Geometry check sheet. Reference: the model listing, model coordinates, mm. Round coordinates to 2 decimals unless told otherwise and drop trailing zeros. Order: outer loops, then holes, each group sorted by start corner. A loop starts at its lowest first (then second) coordinate and runs counter-clockwise, first axis right, second up.
(1) Sectioned sample at B-B (z = -23.6). Record the boundary of the cut face in (x, y).
(2) Go/stop test with flat-tipped pins: pin 1 (4 mm diameter, centred on y = 6.5, z = 106, fed in from +X); pin 2 (2.5 mm diameter, centred on y = 4.5, z = -104.5, fed in from -X); pin 3 (1.9 mm diameter, centred on x = 79, y = 3.5, fed in from -Z). Record where each tip stops, or that it passes through.
(3) Sectioned sample at C-C (y = 7.5). Give the number of separate pieces and of enclosed holes in the cut face, plus the area to 3 significant figures.
(4) Sectioned sample at A-A (x = 70). Record the boundary of the cut face in (y, z).
(5) Sectioned sample at D-D (x = -37.5). Record the boundary of the cut face in (y, z), plus the area to 3 significant figures.
(6) Material ranges on line 1 along Z through (x, y) = (23.5, 2.25); line 2 along X through (y, z) = (6.5, 23.6); line 3 along X through (y, z) = (6.5, -100.5), recorded low to high.
from build123d import *

# Parameters (mm, degrees)
SKETCH1_W            = 260
SKETCH1_H            = 200
EXTRUDE1_DEPTH       = 10
SKETCH3_W            = 20
SKETCH3_H            = 10
EXTRUDE2_DEPTH       = 10
M4_CLEARANCE_HOLE1_D = 4.5
EXTRUDE3_DEPTH       = 10
MIRROR2_COPY_1_DEPTH = 10
MIRROR3_COPY_1_DEPTH = 10
MIRROR3_COPY_2_DEPTH = 10
MIRROR3_COPY_3_DEPTH = 10
SKETCH7_W            = 20
SKETCH7_H            = 10
EXTRUDE4_DEPTH       = 10
LPATTERN1_COUNT      = 2
LPATTERN1_PITCH      = 170
LPATTERN1_COUNT_DIR2 = 2
LPATTERN1_PITCH_DIR2 = 210
EXTRUDE5_DEPTH       = 10
MIRROR5_COPY_1_DEPTH = 10
EXTRUDE6_DEPTH       = 10
MIRROR7_COPY_1_DEPTH = 10
SKETCH11_R           = 19.05
SKETCH11_R_2         = 2.75
CUT_EXTRUDE2_DEPTH   = 10


with BuildPart() as part:
    # Sketch1 → Extrude1 (new body)
    with BuildSketch(Plane(origin=(0, 0, 0), x_dir=(1, 0, 0), z_dir=(0, 1, 0))):
        Rectangle(SKETCH1_W, SKETCH1_H)
    extrude(amount=EXTRUDE1_DEPTH)

    # Sketch3 → Extrude2 (cut)
    with BuildSketch(Plane(origin=(0, 10, 0), x_dir=(1, 0, 0), z_dir=(0, 1, 0))):
        with Locations((-105, 45)):
            Rectangle(SKETCH3_W, SKETCH3_H)
        with Locations((105, 45)):
            Rectangle(SKETCH3_W, SKETCH3_H)
        with Locations((-65, 45)):
            Rectangle(SKETCH3_W, SKETCH3_H)
        with Locations((65, 45)):
            Rectangle(SKETCH3_W, SKETCH3_H)
    extrude(amount=-EXTRUDE2_DEPTH, mode=Mode.SUBTRACT)

    # M4 Clearance Hole1 (through all)
    with Locations(Plane(origin=(0, 10, 0), x_dir=(1, 0, 0), z_dir=(0, 1, 0))):
        with Locations((-85, 45), (85, 45)):
            Hole(M4_CLEARANCE_HOLE1_D / 2)

    # Sketch6 → Extrude3 (cut)
    with BuildSketch(Plane(origin=(0, 10, 0), x_dir=(1, 0, 0), z_dir=(0, 1, 0))):
        with BuildLine():
            Line((-113.5, 50), (-115, 50))
            Line((-115, 50), (-115, 48.5))
            ThreePointArc((-115, 48.5), (-116.060660172, 51.060660172), (-113.5, 50))
        make_face()
        with BuildLine():
            Line((-113.5, 40), (-115, 40))
            Line((-115, 40), (-115, 41.5))
            ThreePointArc((-115, 41.5), (-116.060660172, 38.939339828), (-113.5, 40))
        make_face()
    extrude3 = extrude(amount=-EXTRUDE3_DEPTH, mode=Mode.SUBTRACT)

    # Mirror1: Extrude3 across plane
    add(extrude3.mirror(Plane(origin=(-105, 0, 0), x_dir=(0, 0, 1), z_dir=(1, 0, 0))), mode=Mode.SUBTRACT)

    # Mirror2: Extrude3 across plane
    add(extrude3.mirror(Plane.ZY.offset(85)), mode=Mode.SUBTRACT)

    # Mirror2 copy 1 sketch → Mirror2 copy 1 (cut)
    with BuildSketch(Plane(origin=(40, 10, 0), x_dir=(1, 0, 0), z_dir=(0, 1, 0))):
        with BuildLine():
            Line((-113.5, 50), (-115, 50))
            Line((-115, 50), (-115, 48.5))
            ThreePointArc((-115, 48.5), (-116.060660172, 51.060660172), (-113.5, 50))
        make_face()
        with BuildLine():
            Line((-113.5, 40), (-115, 40))
            Line((-115, 40), (-115, 41.5))
            ThreePointArc((-115, 41.5), (-116.060660172, 38.939339828), (-113.5, 40))
        make_face()
    extrude(amount=-MIRROR2_COPY_1_DEPTH, mode=Mode.SUBTRACT)

    # Mirror3: Extrude3 across plane
    add(extrude3.mirror(Plane(origin=(0, 0, 0), x_dir=(0, 0, 1), z_dir=(1, 0, 0))), mode=Mode.SUBTRACT)

    # Mirror3 copy 1 sketch → Mirror3 copy 1 (cut)
    with BuildSketch(Plane(origin=(210, 10, 0), x_dir=(1, 0, 0), z_dir=(0, 1, 0))):
        with BuildLine():
            Line((-113.5, 50), (-115, 50))
            Line((-115, 50), (-115, 48.5))
            ThreePointArc((-115, 48.5), (-116.060660172, 51.060660172), (-113.5, 50))
        make_face()
        with BuildLine():
            Line((-113.5, 40), (-115, 40))
            Line((-115, 40), (-115, 41.5))
            ThreePointArc((-115, 41.5), (-116.060660172, 38.939339828), (-113.5, 40))
        make_face()
    extrude(amount=-MIRROR3_COPY_1_DEPTH, mode=Mode.SUBTRACT)

    # Mirror3 copy 2 sketch → Mirror3 copy 2 (cut)
    with BuildSketch(Plane(origin=(170, 10, 0), x_dir=(1, 0, 0), z_dir=(0, 1, 0))):
        with BuildLine():
            Line((-113.5, 50), (-115, 50))
            Line((-115, 50), (-115, 48.5))
            ThreePointArc((-115, 48.5), (-116.060660172, 51.060660172), (-113.5, 50))
        make_face()
        with BuildLine():
            Line((-113.5, 40), (-115, 40))
            Line((-115, 40), (-115, 41.5))
            ThreePointArc((-115, 41.5), (-116.060660172, 38.939339828), (-113.5, 40))
        make_face()
    extrude(amount=-MIRROR3_COPY_2_DEPTH, mode=Mode.SUBTRACT)

    # Mirror3 copy 3 sketch → Mirror3 copy 3 (cut)
    with BuildSketch(Plane(origin=(-40, 10, 0), x_dir=(-1, 0, 0), z_dir=(0, 1, 0))):
        with BuildLine():
            Line((-113.5, -50), (-115, -50))
            Line((-115, -50), (-115, -48.5))
            ThreePointArc((-115, -48.5), (-116.060660172, -51.060660172), (-113.5, -50))
        make_face()
        with BuildLine():
            Line((-113.5, -40), (-115, -40))
            Line((-115, -40), (-115, -41.5))
            ThreePointArc((-115, -41.5), (-116.060660172, -38.939339828), (-113.5, -40))
        make_face()
    extrude(amount=-MIRROR3_COPY_3_DEPTH, mode=Mode.SUBTRACT)

    # Sketch7 → Extrude4 (add)
    with BuildSketch(Plane(origin=(0, 10, 0), x_dir=(1, 0, 0), z_dir=(0, 1, 0))):
        with Locations((-105, -105)):
            Rectangle(SKETCH7_W, SKETCH7_H)
        with Locations((-65, -105)):
            Rectangle(SKETCH7_W, SKETCH7_H)
    extrude4 = extrude(amount=-EXTRUDE4_DEPTH)

    # LPattern1: Extrude4 2 × 2
    with Locations(*[(i * LPATTERN1_PITCH, 0, -j * LPATTERN1_PITCH_DIR2) for i in range(LPATTERN1_COUNT) for j in range(LPATTERN1_COUNT_DIR2) if (i, j) != (0, 0)]):
        add(extrude4)

    # Sketch8 → Extrude5 (cut)
    with BuildSketch(Plane(origin=(0, 10, 0), x_dir=(1, 0, 0), z_dir=(0, 1, 0))):
        with BuildLine():
            Line((-116.5, -100), (-115, -100))
            Line((-115, -100), (-115, -101.5))
            ThreePointArc((-115, -101.5), (-113.939339828, -98.939339828), (-116.5, -100))
        make_face()
        with BuildLine():
            Line((-95, -101.5), (-95, -100))
            Line((-95, -100), (-93.5, -100))
            ThreePointArc((-93.5, -100), (-96.060660172, -98.939339828), (-95, -101.5))
        make_face()
        with BuildLine():
            Line((-75, -100), (-75, -101.5))
            ThreePointArc((-75, -101.5), (-73.939339828, -98.939339828), (-76.5, -100))
            Line((-76.5, -100), (-75, -100))
        make_face()
        with BuildLine():
            Line((-55, -101.5), (-55, -100))
            Line((-55, -100), (-53.5, -100))
            ThreePointArc((-53.5, -100), (-56.060660172, -98.939339828), (-55, -101.5))
        make_face()
    extrude5 = extrude(amount=-EXTRUDE5_DEPTH, mode=Mode.SUBTRACT)

    # Mirror4: Extrude5 across plane
    add(extrude5.mirror(Plane(origin=(0, 0, 0), x_dir=(0, 0, 1), z_dir=(1, 0, 0))), mode=Mode.SUBTRACT)

    # Mirror5: Extrude5 across plane
    add(extrude5.mirror(Plane.XY), mode=Mode.SUBTRACT)

    # Mirror5 copy 1 sketch → Mirror5 copy 1 (cut)
    with BuildSketch(Plane(origin=(0, 10, 0), x_dir=(-1, 0, 0), z_dir=(0, 1, 0))):
        with BuildLine():
            Line((-116.5, -100), (-115, -100))
            Line((-115, -100), (-115, -101.5))
            ThreePointArc((-115, -101.5), (-113.939339828, -98.939339828), (-116.5, -100))
        make_face()
        with BuildLine():
            Line((-95, -101.5), (-95, -100))
            Line((-95, -100), (-93.5, -100))
            ThreePointArc((-93.5, -100), (-96.060660172, -98.939339828), (-95, -101.5))
        make_face()
        with BuildLine():
            Line((-75, -100), (-75, -101.5))
            ThreePointArc((-75, -101.5), (-73.939339828, -98.939339828), (-76.5, -100))
            Line((-76.5, -100), (-75, -100))
        make_face()
        with BuildLine():
            Line((-55, -101.5), (-55, -100))
            Line((-55, -100), (-53.5, -100))
            ThreePointArc((-53.5, -100), (-56.060660172, -98.939339828), (-55, -101.5))
        make_face()
    extrude(amount=-MIRROR5_COPY_1_DEPTH, mode=Mode.SUBTRACT)

    # Sketch9 → Extrude6 (cut)
    with BuildSketch(Plane(origin=(0, 10, 0), x_dir=(1, 0, 0), z_dir=(0, 1, 0))):
        Polygon((-87.25, -100), (-87.25, -92), (-88.625, -92), (-88.625, -88.3), (-87.25, -88.3), (-87.25, -84), (-82.75, -84), (-82.75, -88.3), (-81.375, -88.3), (-81.375, -92), (-82.75, -92), (-82.75, -100), align=None)
    extrude6 = extrude(amount=-EXTRUDE6_DEPTH, mode=Mode.SUBTRACT)

    # Mirror6: Extrude6 across plane
    add(extrude6.mirror(Plane(origin=(0, 0, 0), x_dir=(0, 0, 1), z_dir=(1, 0, 0))), mode=Mode.SUBTRACT)

    # Mirror7: Extrude6 across plane
    add(extrude6.mirror(Plane.XY), mode=Mode.SUBTRACT)

    # Mirror7 copy 1 sketch → Mirror7 copy 1 (cut)
    with BuildSketch(Plane(origin=(0, 10, 0), x_dir=(-1, 0, 0), z_dir=(0, 1, 0))):
        Polygon((-87.25, -100), (-87.25, -92), (-88.625, -92), (-88.625, -88.3), (-87.25, -88.3), (-87.25, -84), (-82.75, -84), (-82.75, -88.3), (-81.375, -88.3), (-81.375, -92), (-82.75, -92), (-82.75, -100), align=None)
    extrude(amount=-MIRROR7_COPY_1_DEPTH, mode=Mode.SUBTRACT)

    # Sketch11 → Cut-Extrude2 (cut)
    with BuildSketch(Plane(origin=(-130, 0, 110), x_dir=(0, 0, 1), z_dir=(0, -1, 0))):
        with Locations(Location((-110, -130, 0), (0, 0, 180))):
            Circle(SKETCH11_R)
        with Locations(Location((-133.6, -106.4, 0), (0, 0, 180))):
            Circle(SKETCH11_R_2)
        with Locations(Location((-133.6, -153.6, 0), (0, 0, 180))):
            Circle(SKETCH11_R_2)
        with Locations(Location((-86.4, -153.6, 0), (0, 0, 180))):
            Circle(SKETCH11_R_2)
        with Locations(Location((-86.4, -106.4, 0), (0, 0, 180))):
            Circle(SKETCH11_R_2)
    extrude(amount=-CUT_EXTRUDE2_DEPTH, mode=Mode.SUBTRACT)


solid = part.part
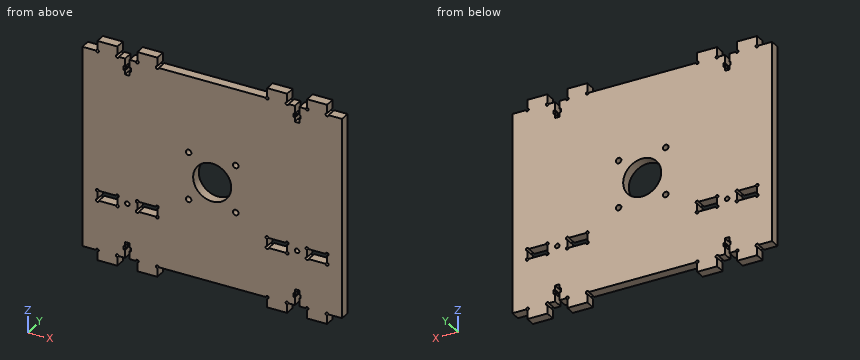
Answer below:
1. outline: (-130, 0) - (-26.35, 0) - (-26.35, 10) - (-130, 10) - close; (-20.85, 0) - (20.85, 0) - (20.85, 10) - (-20.85, 10) - close; (26.35, 0) - (130, 0) - (130, 10) - (26.35, 10) - close
2. pin 1: stops at x = 115
2. pin 2: stops at x = -115
2. pin 3: stops at z = -100
3. separate pieces: 1
3. enclosed holes: 11
3. area: 51,000 mm2
4. outline: (0, -110) - (10, -110) - (10, -50) - (0, -50) - close; (0, -40) - (10, -40) - (10, 110) - (0, 110) - close
5. outline: (0, -100) - (10, -100) - (10, 100) - (0, 100) - close
5. area: 2,000 mm2
6. line 1: z = -100 to -26.35, -20.85 to 20.85, 26.35 to 100
6. line 2: x = -130 to -26.35, -20.85 to 20.85, 26.35 to 130
6. line 3: x = -113.59 to -96.41, -73.59 to -56.41, 56.41 to 73.59, 96.41 to 113.59
